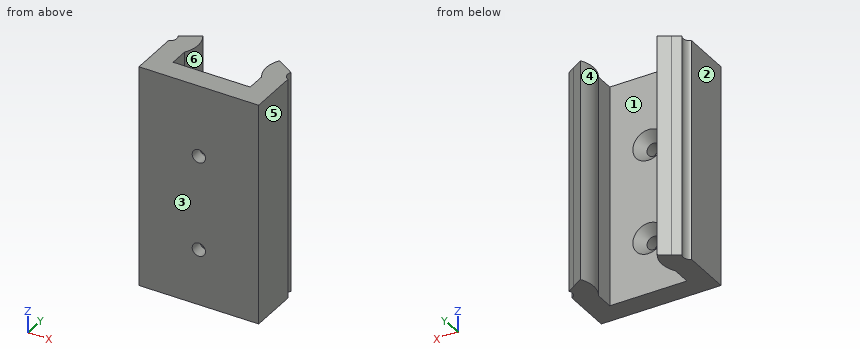
Autodesk Fusion 360 part; units mm, degrees
sketch "Sketch1" plane through (0, 0, 0) normal (0, 0, 1) x (1, 0, 0)
  line L0 (0, 0) -> (17, 0)
  line L1 (0, 0) -> (0, 4)
  line L2 (17, 0) -> (17, 4)
  arc A0 (0, 4) -> (0, 11) centre (-5.625, 7.5) ccw
  arc A1 (17, 11) -> (17, 4) centre (22.625, 7.5) ccw
  line L3 (0, 11) -> (17, 11)
  arc A2 (17.1698, 10.8943) -> (17.2, 4.0576) centre (22.625, 7.5) ccw
  line L4 (17.2, -0.2) -> (17.2, 4.0576)
  line L5 (-0.2, -0.2) -> (17.2, -0.2)
  line L6 (-0.2, -0.2) -> (-0.2, 4.0576)
  arc A3 (-0.2, 4.0576) -> (-0.1698, 10.8943) centre (-5.625, 7.5) ccw
  arc A4 (19.5472, 9.4151) -> (20, 5) centre (22.625, 7.5) ccw
  line L7 (20, -3) -> (20, 5)
  line L8 (-3, -3) -> (20, -3)
  line L9 (-3, -3) -> (-3, 5)
  arc A5 (-3, 5) -> (-2.5472, 9.4151) centre (-5.625, 7.5) ccw
  line L10 (-2.5472, 9.4151) -> (-0.1698, 10.8943)
  line L11 (19.5472, 9.4151) -> (17.1698, 10.8943)
  arc A6 (21.2453, 8.3585) -> (22, 6) centre (22.625, 7.5) ccw
  line L12 (22, -5) -> (22, 6)
  line L13 (-5, -5) -> (22, -5)
  line L14 (-5, -5) -> (-5, 6)
  arc A7 (-5, 6) -> (-4.2453, 8.3585) centre (-5.625, 7.5) ccw
  line L15 (-4.2453, 8.3585) -> (0, 11)
  line L16 (21.2453, 8.3585) -> (17, 11)
  point P0 (0, 11)
  point P1 (17, 11)
  point P2 (1, 7.5)
  point P3 (16, 7.5)
  dimension "d1" = 17
  dimension "d2" = 4
  dimension "d3" = 4
  dimension "d4" = 11
  dimension "d5" = 11
  dimension "d6" = 15
  dimension "d7" = 1
  dimension "d8" = 3.5
  dimension "d9" = 3.5
  dimension "d10" = 0.2
  dimension "d11" = 3
  dimension "d21" = -5
extrude "Extrude1" add sketch "Sketch1" along normal blind 50 contours A2 L4 L5 L6 A3 A4 L7 L8 L9 A5 L10 L11 L15 L16 | A4 L7 L8 L9 A5 A6 L12 L13 L14 A7 L15 L16
sketch "Sketch4" plane through (0, -5, 0) normal (0, -1, 0) x (1, 0, 0)
  line L0 (-5, 0) -> (22, 0)
  line L1 (22, 0) -> (22, 50)
  line L2 (22, 50) -> (-5, 50)
  line L3 (-5, 50) -> (-5, 0)
  circle A0 centre (8.5, 33.9317) radius 1.5
  circle A1 centre (8.5, 12.5947) radius 1.5
  dimension "d25" = 3
  dimension "d26" = 3
  dimension "d27" = 21.337
  dimension "d28" = 13.5
  dimension "d29" = 13.5
extrude "Extrude3" cut sketch "Sketch4" against normal blind 4.8 contours A0 | A1
chamfer "Chamfer4" distance 2 angle 45 2 edges at (7.1015, -0.2, 33.3893) (7.1015, -0.2, 12.0523)
equation "d28 = ( 27 / 2 ) * 1 mm"
equation "d29 = ( 27 / 2 ) * 1 mm"
Input: part model. Units: mm. Frame: model coordinates. Face numbers are marked on the shaded views. A direction names the side the tool comes from. Coordinates: 2 decimals unless noted, no trailing zeros. Write each loop counter-clockwise with the first axis right and the second up, starting at its lowest first coordinate (ties: lowest second). Pieces come first, ordered by that corner, then holes.
1) Section B-B on x = 8.5. Output: boundary loops of the cut face in (y, z).
2) Mould query, pull axis X, two halves, no side actions, for the marked faces 1, 2, 3 and 4. Classes: pulls with the +X half, pulls with the -X half, needs draft (parallel to the pull), parting line crosses it, or undercut.
3) Material intervals for line 1 along Z through (x, y) = (8.5, -3.35); line 2 along X through (y, z) = (2.75, 46.5); line 3 along Y through (x, z) = (15.25, 39.5), sorted ascending.
4) Set-up query: the marked faces 5 and 6. Return all of +Z, -Z, +X, -X, +Y, -Y with unobstructed straight access to the full face (end or side cutting, diameter ignored); none if empty.
5) Section D-D on y = 6.75. Output: boundary loops of the cut face in (x, z), and give its area (3 significant figures).
6) Section A-A on y = 3. Output: boundary loops of the cut face in (x, z), and give its area (3 significant figures).
7) Pin query (flat end, axial travel): pin 1 Ø4 at (x, z) = (8.5, 12.59) entering from -Y; pin 2 Ø1.5 at (y, z) = (7.5, 14) entering from +X; pin 3 Ø12 at (x, z) = (2, 37.5) entering from +Y. Return the tip coordinate at first contact, or that it passes through.
Check result:
1. outline: (-5, 0) - (-0.2, 0) - (-0.2, 9.09) - (-2.2, 11.09) - (-5, 11.09) - close; (-5, 14.09) - (-2.2, 14.09) - (-0.2, 16.09) - (-0.2, 30.43) - (-2.2, 32.43) - (-5, 32.43) - close; (-5, 35.43) - (-2.2, 35.43) - (-0.2, 37.43) - (-0.2, 50) - (-5, 50) - close
2. face 1: undercut
2. face 2: pulls with the -X half
2. face 3: needs draft
2. face 4: undercut
3. line 1: z = 0 to 11.09, 14.09 to 32.43, 35.43 to 50
3. line 2: x = -5 to -0.2, 17.2 to 22
3. line 3: y = -5 to -0.2
4. face 5: +Z, -Z, +X, +Y, -Y
4. face 6: +Z, -Z
5. outline: (-4.18, 0) - (0.76, 0) - (0.76, 50) - (-4.18, 50) - close; (16.24, 0) - (21.18, 0) - (21.18, 50) - (16.24, 50) - close
5. area: 494 mm2
6. outline: (-5, 0) - (-0.2, 0) - (-0.2, 50) - (-5, 50) - close; (17.2, 0) - (22, 0) - (22, 50) - (17.2, 50) - close
6. area: 480 mm2
7. pin 1: stops at y = -5
7. pin 2: stops at x = 21.18
7. pin 3: stops at y = 10.89
